Source: CAD feature listing. Evaluate the final solid. Frame: model axes, mm. A direction names the side the tool comes from. Round coordinates to 2 decimals unless told otherwise and drop trailing zeros. Order: outer loops, then holes, each group sorted by start corner. A loop starts at its lowest first (then second) coordinate and runs counter-clockwise, first axis right, second up. Notation, with made-up numbers: M 87.25,-17.75 L 97.25,-17.75 A12 cw 97.25,-4.75 Z; hole C 75.25,-6.5 d2. An arc over 180 degrees is marked long. Use one line per item in the form item = value. Start each with the question number.
Q1. Pull-direction query (Y, two-part tool) for faces 1 (the cylindrical face through (-0.867, 3.905, -4.58)), 2 (the cylindrical face through (0, 2, -4)), 3 (the flat face through (3, -3, 9)); classes: pulls with the +Y half, pulls with the -Y half, needs draft (parallel to the pull), parting line crosses it, or undercut.
Q2. Reachability of faces 4 (the flat face through (2, -4, 0)), 5 (the flat face through (2, -2, 2)), 6 (the flat face through (2.15, -0.05, -10)) from +Z, -Z, +X, -X, +Y, -Y: full face, straight path, thin tool, end or side. Return the list, or none.
Q3. Section D-D (z = 6.5). Return the cut outline in (x, y), plus the area to 3 significant figures.
Q4. Contact query for flat-ended pins moving along their axis: pin 1 (2 mm diameter, centred on y = 3.5, z = 0, fed in from -X); pin 2 (6 mm diameter, centred on y = 5, z = 2.5, fed in from -X); pin 3 (6 mm diameter, centred on x = 3.5, z = 0.5, fed in from +Y); pin 4 (3.5 mm diameter, centred on x = 1.5, y = -1.5, fed in from +Z). Output: stop coordinate, or through.
Q5. Section A-A (y = 0). Return the cut outline in (x, z), plus the area to 3 significant figures.
Q6. Section C-C (z = -4.75). Return the cut outline in (x, y).
Q7. Material intervals for probe 1 along X at (y, z) = (0, -3.75); probe 2 along Y at (x, z) = (0, 3.75), sorted ascending.
from build123d import *

# Parameters (mm, degrees)
F0_R     = 6.25
F1_DEPTH = 9
F2_R     = 3.5
F3_DEPTH = 7
F4_R     = 4
F5_DEPTH = 10
F6_R     = 2
F7_DEPTH = 12
F8_SIZE2 = 0.71
F8_SIZE  = 0.71
F9_SIZE2 = 0.71
F9_SIZE  = 0.71


with BuildPart() as f1:
    # F0 (on Top) → F1 (new body)
    with BuildSketch(Plane.XY):
        Circle(F0_R)
    extrude(amount=F1_DEPTH)

    # F2 (on face) → F3 (cut)
    with BuildSketch(Plane.XY.offset(9)):
        Circle(F2_R)
    extrude(amount=-F3_DEPTH, mode=Mode.SUBTRACT)

    # F4 (on face) → F5 (join)
    with BuildSketch(Plane(origin=(0, 0, 0), x_dir=(1, 0, 0), z_dir=(0, 0, -1))):
        Circle(F4_R)
    extrude(amount=F5_DEPTH)

    # F6 (on face) → F7 (cut)
    with BuildSketch(Plane(origin=(0, 0, -10), x_dir=(1, 0, 0), z_dir=(0, 0, -1))):
        Circle(F6_R)
    extrude(amount=-F7_DEPTH, mode=Mode.SUBTRACT)

    # F8
    f8_edges = [f1.edges().sort_by_distance(p)[0] for p in [
        (-6.25, 0, 0),
    ]]
    chamfer(f8_edges, length=F8_SIZE, length2=F8_SIZE2)

    # F9
    f9_edges = [f1.edges().sort_by_distance(p)[0] for p in [
        (-4, 0, -10),
    ]]
    chamfer(f9_edges, length=F9_SIZE, length2=F9_SIZE2)


solid = f1.part
Results list:
q1.face_1 = parting line crosses it
q1.face_2 = undercut
q1.face_3 = needs draft
q2.face_4 = -Z
q2.face_5 = +Z
q2.face_6 = -Z, +X, -X, +Y, -Y
q3.outline = C 0,0 d12.5; hole C 0,0 d7
q3.area = 84.2 mm2
q4.pin_1 = -5.59
q4.pin_2 = -5.92
q4.pin_3 = 6.23
q4.pin_4 = 9
q5.outline = M -6.25,0.71 L -5.54,0 L -4,0 L -4,-9.29 L -3.29,-10 L -2,-10 L -2,2 L -3.5,2 L -3.5,9 L -6.25,9 Z; M 2,-10 L 3.29,-10 L 4,-9.29 L 4,0 L 5.54,0 L 6.25,0.71 L 6.25,9 L 3.5,9 L 3.5,2 L 2,2 Z
q5.area = 94.5 mm2
q6.outline = C 0,0 d8; hole C 0,0 d4
q7.probe_1 = -4 to -2, 2 to 4
q7.probe_2 = -6.25 to -3.5, 3.5 to 6.25
